from build123d import *

# Parameters (mm, degrees)
SKETCH1_W           = 25.4
SKETCH1_H           = 124
BOSS_EXTRUDE1_DEPTH = 5
SKETCH2_R           = 2.1
CUT_EXTRUDE1_DEPTH  = 35
SKETCH5_W           = 7.5
SKETCH5_H           = 5
SKETCH5_W_2         = 7.9
CUT_EXTRUDE3_DEPTH  = 10
CUT_EXTRUDE4_DEPTH  = 10


with BuildPart() as part:
    # Sketch1 → Boss-Extrude1 (new body)
    with BuildSketch(Plane.XY):
        with Locations((-24.991212543, -48.06789091)):
            Rectangle(SKETCH1_W, SKETCH1_H)
    extrude(amount=BOSS_EXTRUDE1_DEPTH)

    # Sketch2 → Cut-Extrude1 (cut)
    with BuildSketch(Plane.XY.offset(5)):
        with Locations((-24.791212543, -50.06789091)):
            Circle(SKETCH2_R)
        with Locations((-24.791212543, -80.06789091)):
            Circle(SKETCH2_R)
    extrude(amount=-CUT_EXTRUDE1_DEPTH, mode=Mode.SUBTRACT)

    # Sketch5 → Cut-Extrude3 (cut)
    with BuildSketch(Plane(origin=(0, 0, 0), x_dir=(-1, 0, 0), z_dir=(0, 0, -1))):
        with Locations((16.041212543, -107.56789091)):
            Rectangle(SKETCH5_W, SKETCH5_H)
        with Locations((33.741212543, -107.56789091)):
            Rectangle(SKETCH5_W_2, SKETCH5_H)
    extrude(amount=-CUT_EXTRUDE3_DEPTH, mode=Mode.SUBTRACT)

    # Sketch7 → Cut-Extrude4 (cut)
    with BuildSketch(Plane(origin=(0, 0, 0), x_dir=(-1, 0, 0), z_dir=(0, 0, -1))):
        with BuildLine():
            Line((18.691212543, 13.93210909), (31.291212543, 13.93210909))
            ThreePointArc((31.291212543, 13.93210909), (24.991212543, 7.63210909), (18.691212543, 13.93210909))
        make_face()
    extrude(amount=-CUT_EXTRUDE4_DEPTH, mode=Mode.SUBTRACT)


solid = part.part
The listing builds one solid part. Answer for the finished solid, in the listing's coordinates (mm). A direction names the side the tool comes from. Coordinates: 2 decimals unless noted, no trailing zeros. Write each loop counter-clockwise with the first axis right and the second up, starting at its lowest first coordinate (ties: lowest second). Pieces come first, ordered by that corner, then holes. Notation, with made-up numbers: M -35,80 L -13,80 A31 cw -13,113 Z; hole C -11.75,79 d9. An arc over 180 degrees is marked long. Put each result on its own line as item: value. Start each with the question number.
1. For a pull along X with two mould halves and no side action, classify faces 1 (the cylindrical face through (-26.34, -78.65, 2.54)), 2 (the flat face through (-16, -105.068, 2)), 3 (the flat face through (-29.791, -108, 2)) as pulls with the +X half, pulls with the -X half, needs draft (parallel to the pull), parting line crosses it, or undercut.
2. Consider line 1 (Y direction, x = -16.5, z = 3.45); line 2 (Y direction, x = -27.25, z = 2.7). Determine where each line is inside the solid, lowest interval first. Write a range as from..to.
3. A flat-ended cylindrical pin translates along its axis: P1, Ø2.5, axis at x = -17.5, z = 3, coming from the -Y side. Find the tip coordinate at first contact, or state that the pin passes through.
4. A cutting plane is placed at B-B on z = 2.4. Write down the section's boundary in (x, y).
5. A cutting plane is placed at C-C on x = -14.5. Write down the section's boundary in (y, z), then the cut area to 3 significant figures.
6. Which of the six approach directions +Z, -Z, +X, -X, +Y, -Y give full straight-line access (tool end or side, diameter ignored) to faces 4 (the flat face through (-19.791, -108, 2)), 5 (the flat face through (-25, -47, 5)), 6 (the flat face through (-34, -105.068, 2))?
7. A cutting plane is placed at A-A on x = -24.5. Write down the section's boundary in (y, z), then the cut area to 3 significant figures.
Resolved:
1. face 1: undercut
1. face 2: needs draft
1. face 3: pulls with the -X half
2. line 1: y = -105.07..13.93
2. line 2: y = -110.07..8.05
3. P1: stops at y = -105.07
4. outline: M -37.69,-105.07 L -29.79,-105.07 L -29.79,-110.07 L -19.79,-110.07 L -19.79,-105.07 L -12.29,-105.07 L -12.29,13.93 L -18.69,13.93 A6.3 cw -31.29,13.93 L -37.69,13.93 Z; hole C -24.79,-80.07 d4.2; hole C -24.79,-50.07 d4.2
5. outline: M -105.07,0 L 13.93,0 L 13.93,5 L -105.07,5 Z
5. area: 595 mm2
6. face 4: +Z, -Z, +X, -Y
6. face 5: +Z, +X, -X, +Y, -Y
6. face 6: +Z, -Z, -X, -Y
7. outline: M -110.07,0 L -82.15,0 L -82.15,5 L -110.07,5 Z; M -77.99,0 L -52.15,0 L -52.15,5 L -77.99,5 Z; M -47.99,0 L 7.65,0 L 7.65,5 L -47.99,5 Z
7. area: 547 mm2
